Build history of the part. All positions in model axes, mm. A direction names the side the tool comes from. Give positions to 0.01 mm unless a question says otherwise; leave off trailing zeros. Loops run counter-clockwise (first coordinate to the right, second up) from the corner with the lowest first, then second, coordinate; pieces in that order, holes last. Notation, with made-up numbers: (-38.5, -39.75) -> (-8.5, -39.75) arc R13 ccw to (-8.5, -19.75) -> close; hole circle Ø3 at (-35.75, -27.5). An arc over 180 degrees is marked (long way). Answer as a JSON object with one key per item and string values. Group by question number.
Q1. Band-saw the part on B-B, the plane x = 0. Write the cut outline in (y, z).
Q2. Band-saw the part on A-A, the plane z = 0. Write the cut outline in (x, y).
Q3. Band-saw the part on D-D, the plane z = -40.5. Write the cut outline in (x, y).
Q4. Drop a flat-ended pin along its axis: pin 1 (1.5 mm diameter, centred on y = 1, z = -29.5, fed in from -X). Give the stop position or say it passes through.
Q5. Tool access for faces 5 (the flat face through (-73, 2, -68.262)), 6 (the flat face through (73, 2, -68.262)), 7 (the flat face through (-1, 4.762, -17)): list every direction of +Z, -Z, +X, -X, +Y, -Y with a clear straight run to the whole face (end or side of a thin tool).
Q6. Two-plate mould, pull along X, no slides. Class faces 1 (the flat face through (73, 2, 68.262)), 2 (the flat face through (-71.438, 2, -1)), 3 (the cylindrical face through (1.89, 2.35, 1.45)), 4 (the flat face through (71.438, 2, 1)): pulls with the +X half, pulls with the -X half, needs draft (parallel to the pull), parting line crosses it, or undercut.
Q7. Wall check: probe 1 along Z at (x, y) = (0, 1.95); probe 2 along X at (y, z) = (1.95, 19). Give the ranges that are in metal, low to high. Write a range as from..to.
from build123d import *

# Parameters (mm, degrees)
BOSS_EXTRUDE1_DEPTH            = 4.7625
F_3_16_0_1875_DIAMETER_HOLE1_D = 4.7625
FILLET1_R                      = 1.5875


with BuildPart() as part:
    # Sketch1 → Boss-Extrude1 (new body)
    with BuildSketch(Plane(origin=(0, 0, 0), x_dir=(1, 0, 0), z_dir=(0, 1, 0))):
        Polygon((-71.4375, -71.4375), (71.4375, -71.4375), (76.2, -71.4375), (76.2, -68.2625), (71.4375, -68.2625), (71.4375, 68.2625), (76.2, 68.2625), (76.2, 71.4375), (71.4375, 71.4375), (-71.4375, 71.4375), (-76.2, 71.4375), (-76.2, 68.2625), (-71.4375, 68.2625), (-71.4375, -68.2625), (-76.2, -68.2625), (-76.2, -71.4375), align=None)
    extrude(amount=BOSS_EXTRUDE1_DEPTH)

    # 3/16 (0.1875) Diameter Hole1 (through all)
    with Locations(Plane(origin=(0, 4.7625, 0), x_dir=(1, 0, 0), z_dir=(0, 1, 0))):
        with Locations((0, 0)):
            Hole(F_3_16_0_1875_DIAMETER_HOLE1_D / 2)

    # Fillet1
    fillet1_edges = [part.edges().sort_by_distance(p)[0] for p in [
        (-76.2, 2.38125, 71.4375),
        (-76.2, 2.38125, 68.2625),
        (76.2, 2.38125, 71.4375),
        (76.2, 2.38125, 68.2625),
        (76.2, 2.38125, -68.2625),
        (76.2, 2.38125, -71.4375),
        (-76.2, 2.38125, -68.2625),
        (-76.2, 2.38125, -71.4375),
    ]]
    fillet(fillet1_edges, radius=FILLET1_R - 0.0001)  # a hair under: the kernel refuses the full size


solid = part.part
Worked answers:
{
 "1": {"outline": "(0, -71.44) -> (4.76, -71.44) -> (4.76, -2.38) -> (0, -2.38) -> close; (0, 2.38) -> (4.76, 2.38) -> (4.76, 71.44) -> (0, 71.44) -> close"},
 "2": {"outline": "(-71.44, 0) -> (-2.38, 0) -> (-2.38, 4.76) -> (-71.44, 4.76) -> close; (2.38, 0) -> (71.44, 0) -> (71.44, 4.76) -> (2.38, 4.76) -> close"},
 "3": {"outline": "(-71.44, 0) -> (71.44, 0) -> (71.44, 4.76) -> (-71.44, 4.76) -> close"},
 "4": {"pin 1": "x = -71.44"},
 "5": {"face 5": "-X, +Y, -Y", "face 6": "+X, +Y, -Y", "face 7": "+Z, -Z, +X, -X, +Y"},
 "6": {"face 1": "needs draft", "face 2": "pulls with the -X half", "face 3": "undercut", "face 4": "pulls with the +X half"},
 "7": {"probe 1": "-71.44..-2.38, 2.38..71.44", "probe 2": "-71.44..71.44"}
}
